from build123d import *

# Parameters (mm, degrees)
CROQUIS4_W            = 3.5
CROQUIS4_H            = 1
CORTAR_EXTRUIR1_DEPTH = 1


with BuildPart() as part:
    # Croquis3 → Revolución1 (revolve)
    with BuildSketch(Plane(origin=(0, 0, 0), x_dir=(0, 0, -1), z_dir=(1, 0, 0)), mode=Mode.PRIVATE) as revoluci_n1_sk:
        Polygon((0, 0), (0, 2.5), (-2, 2.5), (-2, 2), (-2.5, 2), (-2.5, 2.5), (-3.5, 2.5), (-3.5, 2), (-6.5, 2), (-6.5, 1.095516127), (-9.5, 0.125), (-9.5, 0), align=None)
    revolve(revoluci_n1_sk.sketch.rotate(Axis((0, 0, 9.5), (0, 0, -1)), 180), axis=Axis((0, 0, 9.5), (0, 0, -1)))

    # Croquis4 → Cortar-Extruir1 (cut)
    with BuildSketch(Plane(origin=(0, 0, 0), x_dir=(-1, 0, 0), z_dir=(0, 0, -1))):
        Rectangle(CROQUIS4_W, CROQUIS4_H)
    extrude(amount=-CORTAR_EXTRUIR1_DEPTH, mode=Mode.SUBTRACT)


solid = part.part
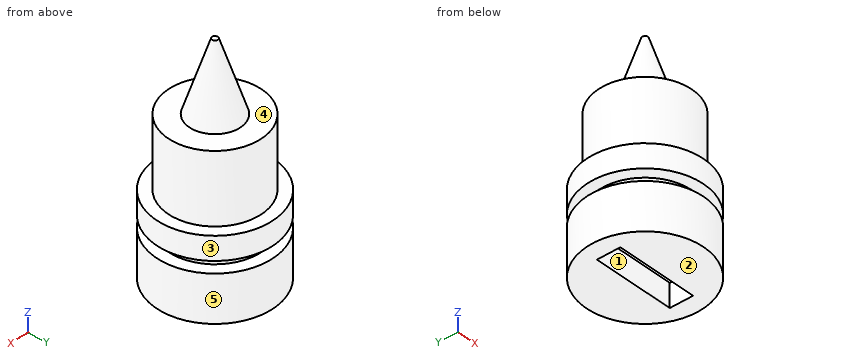
Geometry check sheet. Reference: the model listing, model coordinates, mm. Face numbers are marked on the shaded views. A direction names the side the tool comes from. Give positions to 0.01 mm unless a question says otherwise; leave off trailing zeros. Loops run counter-clockwise (first coordinate to the right, second up) from the corner with the lowest first, then second, coordinate; pieces in that order, holes last. Notation, with made-up numbers: (33.25, 55.5) -> (60.25, 55.5) arc R28 ccw to (60.25, 81.5) -> close; hole circle Ø2 at (2.5, 21). An arc over 180 degrees is marked (long way). Answer in a Markdown table with one row per item. Add a question column.
1) Cross-section at B-B on x = 0. Record the boundary of the cut face in (y, z) (3 decimals).
2) Cross-section at D-D on y = -1.35. Record the boundary of the cut face in (x, z).
3) Set-up check for the marked faces 4 and 5: record each of +Z, -Z, +X, -X, +Y, -Y from which the full face is reachable in a straight line by a thin tool's end or side.
4) Draft check along Y on the marked faces 1, 2 and 3. Enter one of: pulls with the +Y half, pulls with the -Y half, needs draft (parallel to the pull), parting line crosses it, or undercut.
5) Material ranges on probe 1 along Z at (x, y) = (-1.95, 1.15); probe 2 along Z at (x, y) = (-0.65, 1.3); probe 3 along Z at (x, y) = (1.3, -0.05), recorded low to high. Write a range as from..to.
6) Cross-section at C-C on z = 6.25. Record the boundary of the cut face in (x, y).
7) Gauge pin test, flat ends, axial feed: P1, Ø2.5, axis at x = 0, y = -0.5, coming from the -Z side; P2, Ø2, axis at x = 1.5, z = 3.5, coming from the +Y side; P3, Ø0.5, axis at x = -0.5, y = 0, coming from the -Z side; P4, Ø0.5, axis at x = 0.5, z = 0.5, coming from the -Y side. Record the tip position at first contact, or that the pin passes through.
8) Cross-section at A-A on y = 0. Record the boundary of the cut face in (x, z) (3 decimals), and give its area (3 significant figures).
Outcome:
| question | item | result |
|---|---|---|
| 1 | outline | (-2.5, 0) -> (-0.5, 0) -> (-0.5, 1) -> (0.5, 1) -> (0.5, 0) -> (2.5, 0) -> (2.5, 2) -> (2, 2) -> (2, 2.5) -> (2.5, 2.5) -> (2.5, 3.5) -> (2, 3.5) -> (2, 6.5) -> (1.096, 6.5) -> (0.125, 9.5) -> (-0.125, 9.5) -> (-1.096, 6.5) -> (-2, 6.5) -> (-2, 3.5) -> (-2.5, 3.5) -> (-2.5, 2.5) -> (-2, 2.5) -> (-2, 2) -> (-2.5, 2) -> close |
| 2 | outline | (-2.1, 0) -> (2.1, 0) -> (2.1, 2) -> (1.48, 2) -> (1.48, 2.5) -> (2.1, 2.5) -> (2.1, 3.5) -> (1.48, 3.5) -> (1.48, 6.5) -> (-1.48, 6.5) -> (-1.48, 3.5) -> (-2.1, 3.5) -> (-2.1, 2.5) -> (-1.48, 2.5) -> (-1.48, 2) -> (-2.1, 2) -> close |
| 3 | face 4 | +Z |
| 3 | face 5 | +Z, -Z |
| 4 | face 1 | undercut |
| 4 | face 2 | needs draft |
| 4 | face 3 | parting line crosses it |
| 5 | probe 1 | z = 0..2, 2.5..3.5 |
| 5 | probe 2 | z = 0..6.5 |
| 5 | probe 3 | z = 1..6.5 |
| 6 | outline | circle Ø4 at (0, 0) |
| 7 | P1 | stops at z = 0 |
| 7 | P2 | stops at y = 2.45 |
| 7 | P3 | stops at z = 1 |
| 7 | P4 | stops at y = -2.49 |
| 8 | outline | (-2.5, 0) -> (-1.75, 0) -> (-1.75, 1) -> (1.75, 1) -> (1.75, 0) -> (2.5, 0) -> (2.5, 2) -> (2, 2) -> (2, 2.5) -> (2.5, 2.5) -> (2.5, 3.5) -> (2, 3.5) -> (2, 6.5) -> (1.096, 6.5) -> (0.125, 9.5) -> (-0.125, 9.5) -> (-1.096, 6.5) -> (-2, 6.5) -> (-2, 3.5) -> (-2.5, 3.5) -> (-2.5, 2.5) -> (-2, 2.5) -> (-2, 2) -> (-2.5, 2) -> close |
| 8 | area | 29.2 mm^2 |
